```python
from build123d import *

# Parameters (mm, degrees)
SKETCH1_W                                           = 144
SKETCH1_H                                           = 20
BOSS_EXTRUDE1_DEPTH                                 = 6
CSK_FOR_M6_COUNTERSUNK_FLAT_HEAD_SCREW1_D           = 6
CSK_FOR_M6_COUNTERSUNK_FLAT_HEAD_SCREW1_DEPTH       = 17.5
CSK_FOR_M6_COUNTERSUNK_FLAT_HEAD_SCREW1_CSINK_D     = 13
CSK_FOR_M6_COUNTERSUNK_FLAT_HEAD_SCREW1_CSINK_ANGLE = 90
CSK_FOR_M6_COUNTERSUNK_FLAT_HEAD_SCREW1_TIP         = 1.802581857


with BuildPart() as part:
    # Sketch1 → Boss-Extrude1 (new body)
    with BuildSketch(Plane.XY):
        with Locations((16.335821826, 4.315981806)):
            Rectangle(SKETCH1_W, SKETCH1_H)
    extrude(amount=BOSS_EXTRUDE1_DEPTH)

    # CSK for M6 Countersunk Flat Head Screw1
    with Locations(Plane(origin=(0, 0, 0), x_dir=(-1, 0, 0), z_dir=(0, 0, -1))):
        with Locations((-50.335821826, 4.315981806), (19.664178174, 4.315981806)):
            CounterSinkHole(CSK_FOR_M6_COUNTERSUNK_FLAT_HEAD_SCREW1_D / 2, CSK_FOR_M6_COUNTERSUNK_FLAT_HEAD_SCREW1_CSINK_D / 2, depth=CSK_FOR_M6_COUNTERSUNK_FLAT_HEAD_SCREW1_DEPTH, counter_sink_angle=CSK_FOR_M6_COUNTERSUNK_FLAT_HEAD_SCREW1_CSINK_ANGLE)
            with Locations((0, 0, -(CSK_FOR_M6_COUNTERSUNK_FLAT_HEAD_SCREW1_DEPTH + CSK_FOR_M6_COUNTERSUNK_FLAT_HEAD_SCREW1_TIP / 2))):  # 118° drill point
                Cone(0, CSK_FOR_M6_COUNTERSUNK_FLAT_HEAD_SCREW1_D / 2, CSK_FOR_M6_COUNTERSUNK_FLAT_HEAD_SCREW1_TIP, mode=Mode.SUBTRACT)


solid = part.part
```
Part model, mm, in its own coordinate system. Coordinates: 2 decimals unless noted, no trailing zeros. Loops run counter-clockwise (first coordinate to the right, second up) from the corner with the lowest first, then second, coordinate; pieces in that order, holes last. Notation, with made-up numbers: (-26.5, 18.5) - (-18.5, 18.5) arc R32 ccw to (-18.5, 51.5) - close; hole circle Ø11 at (50.25, 17.5). An arc over 180 degrees is marked (long way). Write item = value, one per line. Start each with the question number.
Item 1: Wall check: L1, parallel to X at y = 6, z = 5.3; L2, parallel to X at y = 5.75, z = 1; L3, parallel to Y at x = -20, z = 3.4. Give the ranges that are in metal, low to high. Write a range as from..to.
Item 2: Flat gauge pins, fed straight in: pin 1 Ø7 at (x, y) = (-19.66, 4.32) entering from -Z; pin 2 Ø9.5 at (x, y) = (50.34, 4.32) entering from -Z. Where does each tip first touch, or does it go through?
Item 3: Cut at B-B, the plane y = 3. State how many separate pieces and enclosed holes the cut face has, and give its area (3 significant figures).
Item 4: Cut at A-A, the plane z = 4.95. Give the cut face in (x, y).
Item 5: Mould opens along X. For faces 1 (the cylindrical face through (53.197, 5.217, 4.768)), 2 (the flat face through (-55.664, 4, 3)), 3 (the flat face through (15, 4, 6)), 4 (the flat face through (88.336, 4, 3)) say: released by +X, released by -X, zero draft, split by the parting line, or undercut.
The answers:
q1.L1 = -55.66..-22.15, -17.18..47.85, 52.82..88.34
q1.L2 = -55.66..-24.97, -14.35..45.03, 55.65..88.34
q1.L3 = -5.68..1.23, 7.4..14.32
q2.pin_1 = 2.99
q2.pin_2 = 1.74
q3.separate_pieces = 3
q3.enclosed_holes = 0
q3.area = 773 mm2
q4.outline = (-55.66, -5.68) - (88.34, -5.68) - (88.34, 14.32) - (-55.66, 14.32) - close; hole circle Ø6 at (-19.66, 4.32); hole circle Ø6 at (50.34, 4.32)
q5.face_1 = undercut
q5.face_2 = released by -X
q5.face_3 = zero draft
q5.face_4 = released by +X
